Build history of the part. All positions in model axes, mm. Face numbers are marked on the shaded views. A direction names the side the tool comes from. Give positions to 0.01 mm unless a question says otherwise; leave off trailing zeros. Loops run counter-clockwise (first coordinate to the right, second up) from the corner with the lowest first, then second, coordinate; pieces in that order, holes last.
1) Band-saw the part on A-A on z = 9.75. List the corners of the cut face in (x, y), then the cut area to 3 significant figures.
2) 3-axis set-ups, long thin cutter, end or side, ignore diameter. For the marked faces 1 and 2: which of +Z, -Z, +X, -X, +Y, -Y reach the whole face in a straight line?
3) Flat gauge pins, fed straight in: P1, Ø3, axis at y = 0, z = 4.5, coming from the +X side; P2, Ø3, axis at x = 0, z = 7.5, coming from the +Y side; P3, Ø1.2, axis at x = 0, y = 0, coming from the -Z side; P4, Ø1.5, axis at y = 1.5, z = 13, coming from the +X side. Where does each tip first touch, or does it go through?
4) Wall check: line 1 (Y direction, x = 1.85, z = 0.5); line 2 (Y direction, x = 0.15, z = 13.5); line 3 (Z direction, x = -1.25, y = -0.95). Give the ranges that are in metal, low to high.
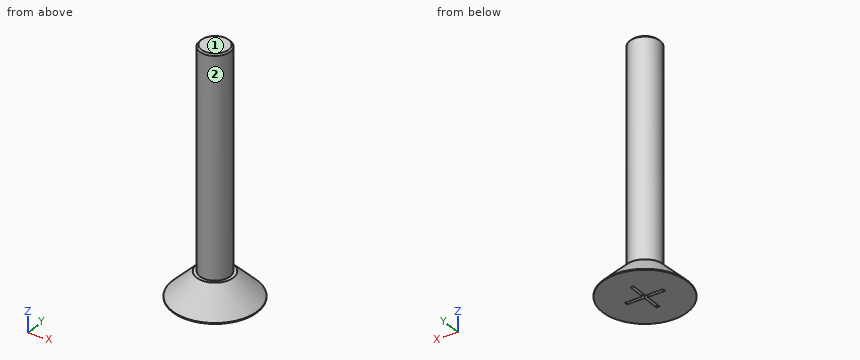
```python
from build123d import *

# Parameters (mm, degrees)
BOX_W             = 0.2
BOX_H             = 2.5
BOX_DEPTH         = 0.5
BOX001_W          = 2.5
BOX001_H          = 0.2
BOX001_DEPTH      = 0.5
CYLINDER_R        = 2.8
CYLINDER_DEPTH    = 1.65
CYLINDER001_R     = 1
CYLINDER001_DEPTH = 16
CHAMFER_SIZE      = 1.59
CHAMFER001_SIZE   = 0.1


with BuildPart() as obj1:
    # Box → Box (new body)
    with BuildSketch(Plane(origin=(-0.1, -1.25, 0), x_dir=(1, 0, 0), z_dir=(0, 0, 1))):
        with Locations((0.1, 1.25)):
            Rectangle(BOX_W, BOX_H)
    extrude(amount=BOX_DEPTH)


with BuildPart() as fusion:
    # Box001 → Box001 (new body)
    with BuildSketch(Plane(origin=(-1.25, -0.1, 0), x_dir=(1, 0, 0), z_dir=(0, 0, 1))):
        with Locations((1.25, 0.1)):
            Rectangle(BOX001_W, BOX001_H)
    extrude(amount=BOX001_DEPTH)

    # Fusion: union obj1
    add(obj1.part)


with BuildPart() as zylinder:
    # Cylinder → Cylinder (new body)
    with BuildSketch(Plane.XY):
        Circle(CYLINDER_R)
    extrude(amount=CYLINDER_DEPTH)


with BuildPart() as screw:
    # Cylinder001 → Cylinder001 (new body)
    with BuildSketch(Plane.XY.offset(0.1)):
        Circle(CYLINDER001_R)
    extrude(amount=CYLINDER001_DEPTH)

    # Fusion001: union Zylinder
    add(zylinder.part)

    # Cut: cut Fusion
    add(fusion.part, mode=Mode.SUBTRACT)

    # Chamfer
    chamfer_edges = [screw.edges().sort_by_distance(p)[0] for p in [
        (-2.8, 0, 1.65),
    ]]
    chamfer(chamfer_edges, length=CHAMFER_SIZE)

    # Chamfer001
    chamfer001_edges = [screw.edges().sort_by_distance(p)[0] for p in [
        (-1, 0, 16.1),
    ]]
    chamfer(chamfer001_edges, length=CHAMFER001_SIZE)


solid = screw.part
```
Findings below:
1. outline: circle Ø2 at (0, 0)
1. area: 3.14 mm2
2. face 1: +Z, +X, -X, +Y, -Y
2. face 2: +Z
3. P1: stops at x = 1
3. P2: stops at y = 1
3. P3: stops at z = 0
3. P4: stops at x = 0.66
4. line 1: y = -1.47 to 1.47
4. line 2: y = -0.99 to 0.99
4. line 3: z = 0 to 1.29
